Can you work these out from the model? Positions are in its coordinate system, mm. Face numbers are marked on the shaded views. A direction names the side the tool comes from. Coordinates: 2 decimals unless noted, no trailing zeros. Loops run counter-clockwise (first coordinate to the right, second up) from the corner with the lowest first, then second, coordinate; pieces in that order, holes last. Notation, with made-up numbers: M 57.5,15 L 104.5,15 A19 ccw 104.5,46 Z; hole C 2,-0.5 d11. An arc over 180 degrees is marked long. Answer as a JSON object with one key per item and string values. Group by question number.
Item 1: Suppose I cut it at C-C (y = 56). Write out the boundary of the cut face in (x, z), then the cut area to 3 significant figures.
Item 2: We'd pull the mould along Y, two halves only. Please class the marked faces 6, 7 and 8: +Y half, -Y half, draft (parallel to the pull), parting line (faces both ways), or undercut.
Item 3: I'm going to push flat-ended pins straight in: pin 1 Ø1.6 at (x, y) = (12.5, 40) entering from +Z; pin 2 Ø10 at (x, z) = (-4, -28.5) entering from +Y; pin 3 Ø4 at (x, y) = (12.5, 46) entering from -Z; pin 4 Ø10.5 at (x, z) = (-2, 28) entering from +Y. Where does each tip first touch, or does it pass through?
Item 4: Suppose I cut it at B-B (x = -6.5). Write out the boundary of the cut face in (y, z).
Item 5: Which directions (+Z, -Z, +X, -X, +Y, -Y) give clear straight access to the entire face, cutting with the end or side of a thin tool? Please do the marked faces 1, 2, 3, 4 and 5.
Item 6: Suppose I cut it at D-D (x = -12). Write out the boundary of the cut face in (y, z).
Item 7: Suppose I cut it at A-A (y = 1). Write out the boundary of the cut face in (x, z), then the cut area to 3 significant figures.
Item 8: If I drill on line 1 (Z direction, x = -0.5, y = -2); line 2 (X direction, y = -0.5, z = 52); line 3 (Z direction, x = 0, y = -8), over which ranges is the centre line in solid material (lowest first)?
```python
from build123d import *

# Parameters (mm, degrees)
SKETCH4_W             = 31.4
SKETCH4_H             = 31.4
SKETCH4_W_2           = 25.4
SKETCH4_H_2           = 25.4
BOSS_EXTRUDE3_DEPTH   = 30
SKETCH5_W             = 31.4
SKETCH5_H             = 31.4
BOSS_EXTRUDE4_DEPTH   = 5
SKETCH6_W             = 31.4
SKETCH6_H             = 8
BOSS_EXTRUDE5_DEPTH   = 5
BOSS_EXTRUDE6_DEPTH   = 8
SKETCH8_R             = 9.5
BOSS_EXTRUDE7_DEPTH   = 8
SKETCH9_W             = 31.4
SKETCH9_H             = 10
BOSS_EXTRUDE8_DEPTH   = 5
SKETCH10_W            = 31.4
SKETCH10_H            = 10
BOSS_EXTRUDE9_DEPTH   = 11
SKETCH11_W            = 5.2
SKETCH11_H            = 10
BOSS_EXTRUDE10_DEPTH  = 40
BOSS_EXTRUDE11_DEPTH  = 3
SKETCH13_W            = 31.4
SKETCH13_H            = 31.4
CUT_EXTRUDE1_DEPTH    = 31.4
SKETCH14_W            = 31.4
SKETCH14_H            = 31.4
BOSS_EXTRUDE12_DEPTH  = 4
SKETCH16_W            = 31.4
SKETCH16_H            = 8
BOSS_EXTRUDE13_DEPTH  = 15.4
CUT_EXTRUDE3_START    = 8
SKETCH8_2_R           = 9.5
CUT_EXTRUDE3_DEPTH    = 24
SKETCH18_W            = 21
SKETCH18_H            = 13
CUT_EXTRUDE4_DEPTH    = 2
MIRROR2_START         = -15.7
MIRROR2_DEPTH         = 34.4
MIRROR2_START_2       = 12.7
MIRROR2_2_OUTLINE_W   = 5.2
MIRROR2_2_OUTLINE_H   = 13
MIRROR2_2_DEPTH       = 48
MIRROR2_START_3       = -4
MIRROR2_3_OUTLINE_R   = 9.5
MIRROR2_3_DEPTH       = 8
MIRROR2_4_OUTLINE_W   = 31.4
MIRROR2_4_OUTLINE_H   = 10
MIRROR2_4_DEPTH       = 14
MIRROR2_5_OUTLINE_W   = 25.4
MIRROR2_5_OUTLINE_H   = 15.4
MIRROR2_5_DEPTH       = 8
MIRROR2_6_OUTLINE_W   = 21
MIRROR2_6_OUTLINE_H   = 5.4
MIRROR2_6_OUTLINE_W_2 = 25.4
MIRROR2_6_OUTLINE_H_2 = 12
MIRROR2_6_DEPTH       = 6
SKETCH17_W            = 30.8
SKETCH17_H            = 24
CUT_EXTRUDE2_DEPTH    = 31.4


# Read off the part's stored shape, not the designer's step: Mirror2
with BuildPart() as part:
    # Sketch4 → Boss-Extrude3 (new body)
    with BuildSketch(Plane.XY):
        Rectangle(SKETCH4_W, SKETCH4_H)
        Rectangle(SKETCH4_W_2, SKETCH4_H_2, mode=Mode.SUBTRACT)
    extrude(amount=BOSS_EXTRUDE3_DEPTH)

    # Sketch5 → Boss-Extrude4 (add)
    with BuildSketch(Plane.XY.offset(30)):
        Rectangle(SKETCH5_W, SKETCH5_H)
    extrude(amount=BOSS_EXTRUDE4_DEPTH)

    # Sketch6 → Boss-Extrude5 (add)
    with BuildSketch(Plane.XY.offset(35)):
        Rectangle(SKETCH6_W, SKETCH6_H)
    extrude(amount=BOSS_EXTRUDE5_DEPTH)

    # Sketch7 → Boss-Extrude6 (add)
    with BuildSketch(Plane.XZ.offset(4)):
        with BuildLine():
            Line((-15.7, 40), (-15.7, 52))
            ThreePointArc((-15.7, 52), (-11.306601718, 62.606601718), (-0.7, 67))
            Line((-0.7, 67), (0.7, 67))
            ThreePointArc((0.7, 67), (11.306601718, 62.606601718), (15.7, 52))
            Line((15.7, 52), (15.7, 40))
            Line((15.7, 40), (-15.7, 40))
        make_face()
    extrude(amount=-BOSS_EXTRUDE6_DEPTH)

    # Sketch8 → Boss-Extrude7 (add)
    with BuildSketch(Plane.XZ.offset(4)):
        with Locations(Location((0, 52, 0), (0, 0, 180))):
            Circle(SKETCH8_R)
    boss_extrude7 = extrude(amount=BOSS_EXTRUDE7_DEPTH)

    # Mirror1: Boss-Extrude7 across plane
    add(boss_extrude7.mirror(Plane.ZX))

    # Sketch9 → Boss-Extrude8 (add)
    with BuildSketch(Plane(origin=(0, 15.7, 0), x_dir=(1, 0, 0), z_dir=(0, 1, 0))):
        with Locations((0, -27)):
            Rectangle(SKETCH9_W, SKETCH9_H)
    extrude(amount=BOSS_EXTRUDE8_DEPTH)

    # Sketch10 → Boss-Extrude9 (add)
    with BuildSketch(Plane(origin=(0, 15.7, 0), x_dir=(1, 0, 0), z_dir=(0, 1, 0))):
        with Locations((0, -17)):
            Rectangle(SKETCH10_W, SKETCH10_H)
    extrude(amount=BOSS_EXTRUDE9_DEPTH)

    # Sketch11 → Boss-Extrude10 (add)
    with BuildSketch(Plane(origin=(0, 20.7, 0), x_dir=(1, 0, 0), z_dir=(0, 1, 0))):
        with Locations((-13.1, -27)):
            Rectangle(SKETCH11_W, SKETCH11_H)
        with Locations((13.1, -27)):
            Rectangle(SKETCH11_W, SKETCH11_H)
    extrude(amount=BOSS_EXTRUDE10_DEPTH)

    # Sketch12 → Boss-Extrude11 (add)
    with BuildSketch(Plane.XY.offset(32)):
        Polygon((-15.7, 60.7), (-10.5, 60.7), (-10.5, 20.7), (10.5, 20.7), (10.5, 60.7), (15.7, 60.7), (15.7, 15.7), (-15.7, 15.7), align=None)
    extrude(amount=BOSS_EXTRUDE11_DEPTH)

    # Sketch13 → Cut-Extrude1 (cut)
    with BuildSketch(Plane.ZY.offset(15.7)):
        with Locations((15.7, 0)):
            Rectangle(SKETCH13_W, SKETCH13_H)
    extrude(amount=-CUT_EXTRUDE1_DEPTH, mode=Mode.SUBTRACT)

    # Sketch14 → Boss-Extrude12 (add)
    with BuildSketch(Plane(origin=(0, 0, 31.4), x_dir=(-1, 0, 0), z_dir=(0, 0, -1))):
        Rectangle(SKETCH14_W, SKETCH14_H)
    extrude(amount=BOSS_EXTRUDE12_DEPTH)

    # Sketch16 → Boss-Extrude13 (add)
    with BuildSketch(Plane(origin=(0, 0, 27.4), x_dir=(-1, 0, 0), z_dir=(0, 0, -1))):
        with Locations((0, -11.7)):
            Rectangle(SKETCH16_W, SKETCH16_H)
    extrude(amount=BOSS_EXTRUDE13_DEPTH)

    # Sketch8<2> → Cut-Extrude3 (cut)
    with BuildSketch(Plane.XZ.offset(4).offset(CUT_EXTRUDE3_START)):
        with Locations(Location((0, 52, 0), (0, 0, 270))):
            Circle(SKETCH8_2_R)
    extrude(amount=-CUT_EXTRUDE3_DEPTH, mode=Mode.SUBTRACT)

    # Sketch18 → Cut-Extrude4 (cut)
    with BuildSketch(Plane(origin=(0, 20.7, 0), x_dir=(1, 0, 0), z_dir=(0, 1, 0))):
        with Locations((0, -28.5)):
            Rectangle(SKETCH18_W, SKETCH18_H)
    extrude(amount=-CUT_EXTRUDE4_DEPTH, mode=Mode.SUBTRACT)

    # Mirror2 outline → Mirror2 (add)
    with BuildSketch(Plane(origin=(0, 0, 0), x_dir=(1, 0, 0), z_dir=(0, 1, 0)).offset(MIRROR2_START)):
        Polygon((-15.7, 11), (-15.7, -24), (-12.7, -24), (-12.7, 3.4), (12.7, 3.4), (12.7, -24), (15.7, -24), (15.7, 11), align=None)
    extrude(amount=MIRROR2_DEPTH)

    # Mirror2 2 outline → Mirror2 2 (add)
    with BuildSketch(Plane(origin=(0, 0, 0), x_dir=(1, 0, 0), z_dir=(0, 1, 0)).offset(MIRROR2_START_2)):
        with Locations((-13.1, 4.5)):
            Rectangle(MIRROR2_2_OUTLINE_W, MIRROR2_2_OUTLINE_H)
        with Locations((13.1, 4.5)):
            Rectangle(MIRROR2_2_OUTLINE_W, MIRROR2_2_OUTLINE_H)
    extrude(amount=MIRROR2_2_DEPTH)

    # Mirror2 3 outline → Mirror2 3 (add)
    with BuildSketch(Plane(origin=(0, 0, 0), x_dir=(1, 0, 0), z_dir=(0, 1, 0)).offset(MIRROR2_START_3)):
        with BuildLine():
            Line((-15.7, 28), (-15.7, 11))
            Line((-15.7, 11), (15.7, 11))
            Line((15.7, 11), (15.7, 28))
            ThreePointArc((15.7, 28), (11.306601718, 38.606601718), (0.7, 43))
            Line((0.7, 43), (-0.7, 43))
            ThreePointArc((-0.7, 43), (-11.306601718, 38.606601718), (-15.7, 28))
        make_face()
        with Locations((0, 28)):
            Circle(MIRROR2_3_OUTLINE_R, mode=Mode.SUBTRACT)
    extrude(amount=MIRROR2_3_DEPTH)

    # Mirror2 4 outline → Mirror2 4 (add)
    with BuildSketch(Plane(origin=(0, 0, 0), x_dir=(1, 0, 0), z_dir=(0, 1, 0)).offset(MIRROR2_START_2)):
        with Locations((0, -7)):
            Rectangle(MIRROR2_4_OUTLINE_W, MIRROR2_4_OUTLINE_H)
    extrude(amount=MIRROR2_4_DEPTH)

    # Mirror2 5 outline → Mirror2 5 (add)
    with BuildSketch(Plane(origin=(0, 0, 0), x_dir=(1, 0, 0), z_dir=(0, 1, 0)).offset(MIRROR2_START)):
        with Locations((0, -4.3)):
            Rectangle(MIRROR2_5_OUTLINE_W, MIRROR2_5_OUTLINE_H)
    extrude(amount=MIRROR2_5_DEPTH)

    # Mirror2 6 outline → Mirror2 6 (add)
    with BuildSketch(Plane(origin=(0, 0, 0), x_dir=(1, 0, 0), z_dir=(0, 1, 0)).offset(MIRROR2_START_2)):
        with Locations((0, 0.7)):
            Rectangle(MIRROR2_6_OUTLINE_W, MIRROR2_6_OUTLINE_H)
        with Locations((0, -18)):
            Rectangle(MIRROR2_6_OUTLINE_W_2, MIRROR2_6_OUTLINE_H_2)
    extrude(amount=MIRROR2_6_DEPTH)

    # Sketch17 → Cut-Extrude2 (cut)
    with BuildSketch(Plane.ZY.offset(15.7)):
        with Locations((12, 3.7)):
            Rectangle(SKETCH17_W, SKETCH17_H)
    extrude(amount=-CUT_EXTRUDE2_DEPTH, mode=Mode.SUBTRACT)


solid = part.part
```
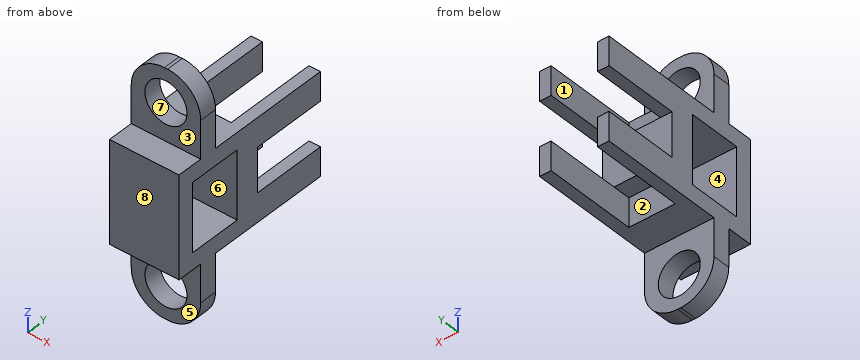
From the geometry:
{
 "1": {"outline": "M -15.7,-11 L -10.5,-11 L -10.5,2 L -15.7,2 Z; M -15.7,22 L -10.5,22 L -10.5,35 L -15.7,35 Z; M 10.5,-11 L 15.7,-11 L 15.7,2 L 10.5,2 Z; M 10.5,22 L 15.7,22 L 15.7,35 L 10.5,35 Z", "area": "270 mm2"},
 "2": {"face 6": "undercut", "face 7": "draft", "face 8": "-Y half"},
 "3": {"pin 1": "z = 35", "pin 2": "through", "pin 3": "z = -11", "pin 4": "y = 18.7"},
 "4": {"outline": "M -15.7,-11 L -4,-11 L -4,-21.07 L 4,-21.07 L 4,-11 L 18.7,-11 L 18.7,2 L 26.7,2 L 26.7,22 L 18.7,22 L 18.7,35 L 4,35 L 4,45.07 L -4,45.07 L -4,35 L -15.7,35 Z; M -4,-41.83 L 4,-41.83 L 4,-34.93 L -4,-34.93 Z; M -4,58.93 L 4,58.93 L 4,65.83 L -4,65.83 Z; hole M -8.3,-3.4 L 15.7,-3.4 L 15.7,27.4 L -8.3,27.4 Z"},
 "5": {"face 1": "+Z, +Y", "face 2": "-Z, +Y", "face 3": "+Z, +X, -X, -Y", "face 4": "+X, -X", "face 5": "-Z, +X, -X, -Y"},
 "6": {"outline": "M -15.7,-11 L -4,-11 L -4,-37.86 L 4,-37.86 L 4,-11 L 60.7,-11 L 60.7,2 L 26.7,2 L 26.7,22 L 60.7,22 L 60.7,35 L 4,35 L 4,61.86 L -4,61.86 L -4,35 L -15.7,35 Z; hole M -8.3,-3.4 L 15.7,-3.4 L 15.7,27.4 L -8.3,27.4 Z"},
 "7": {"outline": "M -15.7,-28 A15 ccw -0.7,-43 L 0.7,-43 A15 ccw 15.7,-28 L 15.7,-3.4 L -15.7,-3.4 Z; M -15.7,27.4 L 15.7,27.4 L 15.7,52 A15 ccw 0.7,67 L -0.7,67 A15 ccw -15.7,52 Z; hole C 0,-28 d19; hole C 0,52 d19", "area": "1,730 mm2"},
 "8": {"line 1": "-43 to -37.49, -18.51 to -3.4, 27.4 to 42.51, 61.49 to 67", "line 2": "-15.7 to -9.5, 9.5 to 15.7", "line 3": "-11 to -3.4, 27.4 to 35"}
}
